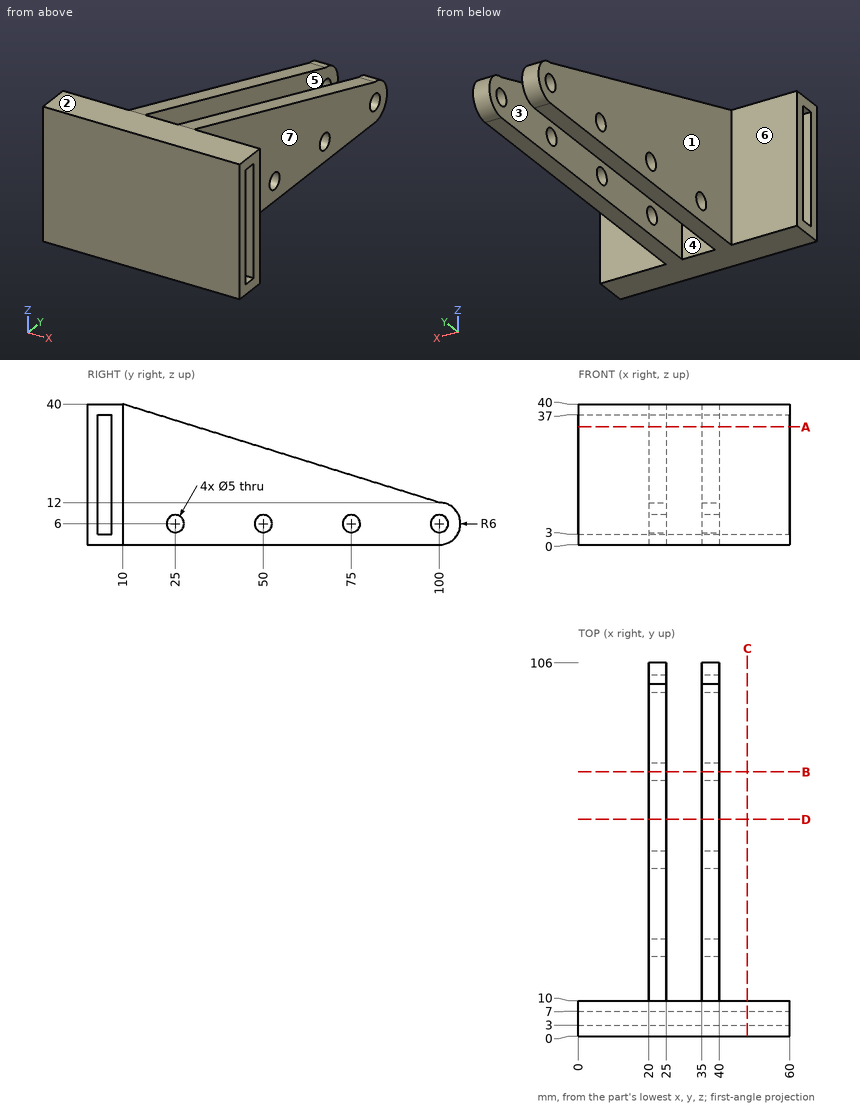
Input: dimensioned drawing with shaded views. Units: mm. Origin: part minimum x, y, z. A direction names the side the tool comes from. Coordinates: 2 decimals unless noted, no trailing zeros. Loops run counter-clockwise (first coordinate to the right, second up) from the corner with the lowest first, then second, coordinate; pieces in that order, holes last. Notation, with made-up numbers: M 21.25,-3 L 80.25,-3 A21 cw 80.25,34 Z; hole C 35.5,84 d7. An arc over 180 degrees is marked long. Use a Markdown table: item, result. Add a question column.
Q1. Section query D-D, the plane y = 61.5. Return loops of the section in (x, z), and give its area (3 significant figures).
Q2. Section query A-A, the plane z = 33.5. Return loops of the section in (x, y), and give its area (3 significant figures).
Q3. Section query C-C, the plane x = 48. Return loops of the section in (y, z).
Q4. Material intervals for L1, parallel to Y at x = 22.15, z = 6; L2, parallel to Y at x = 14, z = 19; L3, parallel to X at y = 73, z = 10.5, sorted ascending.
Q5. Access query for the marked faces 5, 6 and 7. Directions: +Z, -Z, +X, -X, +Y, -Y. A direction counts if a zero-diameter tool reaches every point of the face in a straight line with its end or side. Return the directions, or none.
Q6. Draft query along X for the marked faces 1, 2, 3 and 4. Return one class per face: pulls with the +X half, pulls with the -X half, needs draft (parallel to the pull), parting line crosses it, or undercut.
Q7. First-contact query: pin 1 (12 mm diameter, centred on y = 66, z = 19.5, fed in from +X); pin 2 (4.5 mm diameter, centred on y = 50, z = 6, fed in from -X); pin 3 (6 mm diameter, centred on x = 9, z = 12, fed in from +Y). Flat tips, straight axial feed; report the tip coordinate or a pass-through.
Q8. Section query B-B, the plane y = 75. Return loops of the section in (x, z), and give its area (3 significant figures).
Result:
| question | item | result |
|---|---|---|
| 1 | outline | M 20,0 L 25,0 L 25,23.98 L 20,23.98 Z; M 35,0 L 40,0 L 40,23.98 L 35,23.98 Z |
| 1 | area | 240 mm2 |
| 2 | outline | M 0,0 L 60,0 L 60,3 L 0,3 Z; M 0,7 L 60,7 L 60,10 L 40,10 L 40,30.89 L 35,30.89 L 35,10 L 25,10 L 25,30.89 L 20,30.89 L 20,10 L 0,10 Z |
| 2 | area | 569 mm2 |
| 3 | outline | M 0,0 L 10,0 L 10,40 L 0,40 Z; hole M 3,3 L 7,3 L 7,37 L 3,37 Z |
| 4 | L1 | y = 0 to 3, 7 to 22.5, 27.5 to 47.5, 52.5 to 72.5, 77.5 to 97.5, 102.5 to 106 |
| 4 | L2 | y = 0 to 3, 7 to 10 |
| 4 | L3 | x = 20 to 25, 35 to 40 |
| 5 | face 5 | +Z, -Z, +Y |
| 5 | face 6 | +Z, -Z, -X, +Y |
| 5 | face 7 | +Z, -Z, +X, +Y |
| 6 | face 1 | pulls with the -X half |
| 6 | face 2 | needs draft |
| 6 | face 3 | undercut |
| 6 | face 4 | undercut |
| 7 | pin 1 | stops at x = 40 |
| 7 | pin 2 | passes through |
| 7 | pin 3 | stops at y = 10 |
| 8 | outline | M 20,0 L 25,0 L 25,3.5 L 20,3.5 Z; M 20,8.5 L 25,8.5 L 25,19.78 L 20,19.78 Z; M 35,0 L 40,0 L 40,3.5 L 35,3.5 Z; M 35,8.5 L 40,8.5 L 40,19.78 L 35,19.78 Z |
| 8 | area | 148 mm2 |
